from build123d import *

# Parameters (mm, degrees)
F0_W     = 11
F0_H     = 30
F1_DEPTH = 24
F3_DEPTH = 30.3


with BuildPart() as f1:
    # F0 (on Right) → F1 (new body, symmetric)
    with BuildSketch(Plane.YZ):
        with BuildLine():
            Line((-48.1145605445, 0), (-30, 0))
            ThreePointArc((-30, 0), (-29.4730143031, 5.5983415304), (-27.9105714739, 11))
            Line((-27.9105714739, 11), (-48.1145605445, 11))
            Line((-48.1145605445, 11), (-48.1145605445, 0))
        make_face()
        with Locations((53.3854394555, 26)):
            Rectangle(F0_W, F0_H)
        with BuildLine():
            ThreePointArc((27.9105714739, 11), (29.4730143031, 5.5983415304), (30, 0))
            Line((30, 0), (58.8854394555, 0))
            Line((58.8854394555, 0), (58.8854394555, 11))
            Line((58.8854394555, 11), (47.8854394555, 11))
            Line((47.8854394555, 11), (27.9105714739, 11))
        make_face()
        with BuildLine():
            Line((15.4919333848, 11), (27.9105714739, 11))
            ThreePointArc((27.9105714739, 11), (0, 30), (-27.9105714739, 11))
            Line((-27.9105714739, 11), (-15.4919333848, 11))
            ThreePointArc((-15.4919333848, 11), (0, 19), (15.4919333848, 11))
        make_face()
        with BuildLine():
            Line((19, 0), (30, 0))
            ThreePointArc((30, 0), (29.4730143031, 5.5983415304), (27.9105714739, 11))
            Line((27.9105714739, 11), (15.4919333848, 11))
            ThreePointArc((15.4919333848, 11), (18.1017503893, 5.7729223833), (19, 0))
        make_face()
        with BuildLine():
            ThreePointArc((-27.9105714739, 11), (-29.4730143031, 5.5983415304), (-30, 0))
            Line((-30, 0), (-19, 0))
            ThreePointArc((-19, 0), (-18.1017503893, 5.7729223833), (-15.4919333848, 11))
            Line((-15.4919333848, 11), (-27.9105714739, 11))
        make_face()
    extrude(amount=F1_DEPTH, both=True)

    # F2 (on face) → F3 (cut)
    with BuildSketch(Plane(origin=(0, 58.8854394555, 0), x_dir=(-1, 0, 0), z_dir=(0, 1, 0))):
        with BuildLine():
            ThreePointArc((-6.5, 25), (0, 18.5), (6.5, 25))
            ThreePointArc((6.5, 25), (0, 31.5), (-6.5, 25))
        make_face()
        with BuildLine():
            ThreePointArc((-6.5, 25), (0, 31.5), (6.5, 25))
            Line((6.5, 25), (6.5, 41))
            Line((6.5, 41), (-6.5, 41))
            Line((-6.5, 41), (-6.5, 25))
        make_face()
    extrude(amount=-F3_DEPTH, mode=Mode.SUBTRACT)


solid = f1.part
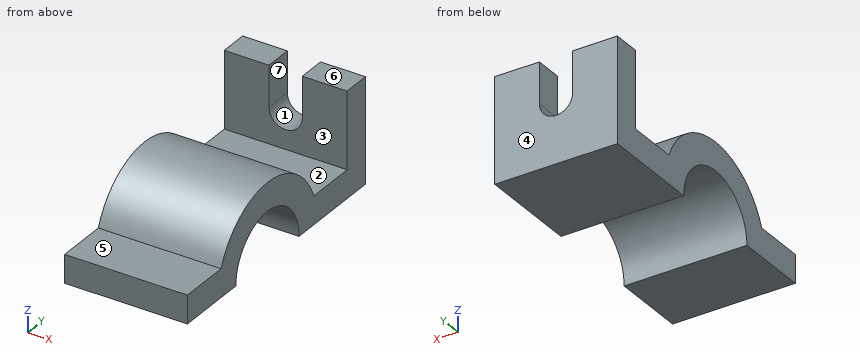
Part model, mm, in its own coordinate system. Face numbers are marked on the shaded views. A direction names the side the tool comes from. Round coordinates to 2 decimals unless told otherwise and drop trailing zeros. Write each loop counter-clockwise with the first axis right and the second up, starting at its lowest first coordinate (ties: lowest second). Pieces come first, ordered by that corner, then holes. Notation, with made-up numbers: M 27,68 L 50,68 A14 cw 50,89 Z; hole C 60,-29.75 d7. An arc over 180 degrees is marked long. Return JSON: item names as keys, results as strings. Group by question number.
(1) Two-plate mould, pull along Y, no slides. Class the marked faces 1, 2, 3 and 4: +Y half, -Y half, draft (parallel to the pull), parting line (faces both ways), or undercut.
(2) Saw through at B-B on z = 34. Write the cut outline in (x, y).
(3) Saw through at A-A on x = 0. Write the cut outline in (y, z), then the cut area to 3 significant figures.
(4) Saw through at D-D on y = -34. Write the cut outline in (x, z), then the cut area to 3 significant figures.
(5) Saw through at C-C on z = 23. Write the cut outline in (x, y).
(6) Drill centre lines: probe 1 along Y at (x, z) = (-8, 16); probe 2 along Z at (x, y) = (-5.5, -36.5); probe 3 along Y at (x, z) = (-13.5, 14.5). Where is each one in solid material? Low to high.
(7) Pin check, flat tips, straight feed: pin 1 Ø2 at (x, y) = (-9, 2.5) entering from +Z; pin 2 Ø15 at (x, z) = (-7.5, 28) entering from -Y; pin 3 Ø22 at (x, y) = (-9.5, 35.5) entering from +Z. Stop position of each tip, or through.
(8) Which spindle directions (+Z, -Z, +X, -X, +Y, -Y) get a long thin tool onto all of the face, cutting with end or side? Do the marked faces 5, 6 and 7. Say none if no direction does.
Returned:
{
 "1": {"face 1": "draft", "face 2": "undercut", "face 3": "undercut", "face 4": "+Y half"},
 "2": {"outline": "M -24,47.89 L -6.5,47.89 L -6.5,58.89 L -24,58.89 Z; M 6.5,47.89 L 24,47.89 L 24,58.89 L 6.5,58.89 Z"},
 "3": {"outline": "M -48.11,0 L -19,0 A19 cw 19,0 L 58.89,0 L 58.89,18.5 L 47.89,18.5 L 47.89,11 L 27.91,11 A30 ccw -27.91,11 L -48.11,11 Z", "area": "1,460 mm²"},
 "4": {"outline": "M -24,0 L 24,0 L 24,11 L -24,11 Z", "area": "528 mm²"},
 "5": {"outline": "M -24,-19.26 L 24,-19.26 L 24,19.26 L -24,19.26 Z; M -24,47.89 L -6.18,47.89 L -6.18,58.89 L -24,58.89 Z; M 6.18,47.89 L 24,47.89 L 24,58.89 L 6.18,58.89 Z"},
 "6": {"probe 1": "-25.38 to -10.25, 10.25 to 25.38, 47.89 to 58.89", "probe 2": "0 to 11", "probe 3": "-26.26 to -12.28, 12.28 to 26.26, 47.89 to 58.89"},
 "7": {"pin 1": "z = 29.96", "pin 2": "y = -21.9", "pin 3": "z = 17.31"},
 "8": {"face 5": "+Z, +X, -X, -Y", "face 6": "+Z, +X, -X, +Y, -Y", "face 7": "+Z, +Y"}
}
